```python
from build123d import *

# Parameters (mm, degrees)
SKETCH1_R           = 16
BASE_EXTRUDE_DEPTH  = 3
EXTRUDE3_DEPTH      = 62
BOSS_EXTRUDE1_DEPTH = 90
SKETCH6_R           = 16
BOSS_EXTRUDE2_DEPTH = 6
SKETCH9_W           = 18
SKETCH9_H           = 30
CUT_EXTRUDE1_DEPTH  = 107.423681603
SKETCH7_R           = 12.5
EXTRUDE4_DEPTH      = 100


with BuildPart() as part:
    # Sketch1 → Base-Extrude (new, symmetric)
    with BuildSketch(Plane.XY):
        Circle(SKETCH1_R)
    extrude(amount=BASE_EXTRUDE_DEPTH, both=True)

    # Sketch2 → Extrude3 (add)
    with BuildSketch(Plane.XY.offset(3)):
        with BuildLine():
            Line((-6, -6.5), (-6, 6.5))
            ThreePointArc((-6, 6.5), (0, 12.5), (6, 6.5))
            Line((6, 6.5), (6, -6.5))
            ThreePointArc((6, -6.5), (0, -12.5), (-6, -6.5))
        make_face()
    extrude(amount=EXTRUDE3_DEPTH)

    # Sketch5 → Boss-Extrude1 (add)
    with BuildSketch(Plane(origin=(0, 0, -3), x_dir=(-1, 0, 0), z_dir=(0, 0, -1))):
        with BuildLine():
            Line((-3, 3), (-3, 10))
            ThreePointArc((-3, 10), (0, 13), (3, 10))
            Line((3, 10), (3, 3))
            Line((3, 3), (10, 3))
            ThreePointArc((10, 3), (13, 0), (10, -3))
            Line((10, -3), (3, -3))
            Line((3, -3), (3, -10))
            ThreePointArc((3, -10), (0, -13), (-3, -10))
            Line((-3, -10), (-3, -3))
            Line((-3, -3), (-10, -3))
            ThreePointArc((-10, -3), (-13, 0), (-10, 3))
            Line((-10, 3), (-3, 3))
        make_face()
    extrude(amount=BOSS_EXTRUDE1_DEPTH)

    # Sketch6 → Boss-Extrude2 (add)
    with BuildSketch(Plane(origin=(0, 0, -93), x_dir=(-1, 0, 0), z_dir=(0, 0, -1))):
        with Locations(Location((0, 0, 0), (0, 0, 180))):
            Circle(SKETCH6_R)
    extrude(amount=BOSS_EXTRUDE2_DEPTH)

    # Sketch9 → Boss-Revolve1 (revolve)
    with BuildSketch(Plane.XY.offset(65), mode=Mode.PRIVATE) as boss_revolve1_sk:
        with Locations((0, 15)):
            Rectangle(SKETCH9_W, SKETCH9_H)
    revolve(boss_revolve1_sk.sketch.rotate(Axis((9, 0, 65), (1, 0, 0)), 180), axis=Axis((9, 0, 65), (1, 0, 0)))

    # Sketch10 → Cut-Extrude1 (cut, through all)
    with BuildSketch(Plane(origin=(9, 0, 0), x_dir=(0, 0, -1), z_dir=(1, 0, 0))):
        with BuildLine():
            Line((-72.483314774, 13), (-57.516685226, 13))
            ThreePointArc((-57.516685226, 13), (-65, -15), (-72.483314774, 13))
        make_face()
    extrude(amount=-CUT_EXTRUDE1_DEPTH, mode=Mode.SUBTRACT)

    # Sketch7 → Extrude4 (add)
    with BuildSketch(Plane(origin=(0, 0, -99), x_dir=(-1, 0, 0), z_dir=(0, 0, -1))):
        Circle(SKETCH7_R)
    extrude(amount=EXTRUDE4_DEPTH)


solid = part.part
```
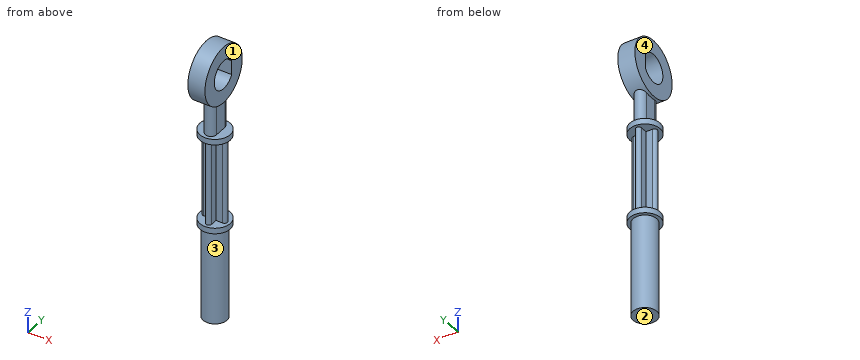
Model file for the job. Use its own axes, mm. Face numbers are marked on the shaded views. A direction names the side the tool comes from. Coordinates: 2 decimals unless noted, no trailing zeros. Write each loop counter-clockwise with the first axis right and the second up, starting at its lowest first coordinate (ties: lowest second). Pieces come first, ordered by that corner, then holes. Notation, with made-up numbers: (54.5, -37) - (103.5, -37) arc R31 ccw to (103.5, -6) - close; hole circle Ø3 at (-13, 62). An arc over 180 degrees is marked (long way). Use a Markdown table: item, result. Add a question column.
Item 1: Drop flat-ended pins along their axis: pin 1 (7.5 mm diameter, centred on x = -7, z = -58, fed in from +Y); pin 2 (18 mm diameter, centred on y = 0, z = 65, fed in from -X); pin 3 (3.5 mm diameter, centred on y = 7.5, z = -32.5, fed in from -X); pin 4 (10.5 mm diameter, centred on y = 1.5, z = 21, fed in from +X). Give the stop position or say it passes through.
Item 2: Band-saw the part on D-D, the plane y = 19. Write the cut outline in (x, z), and give its area (3 significant figures).
Item 3: Band-saw the part on A-A, the plane y = 0. Write the cut outline in (x, z), and give its area (3 significant figures).
Item 4: Band-saw the part on B-B, the plane z = -10. Write the cut outline in (x, y), and give its area (3 significant figures).
Item 5: Drill centre lines: line 1 along Z through (x, y) = (-2, 0); line 2 along Y through (x, z) = (2, 65); line 3 along Z through (x, y) = (-10, 12). Where is each one in solid material? Low to high.
Item 6: 3-axis set-ups, long thin cutter, end or side, ignore diameter. For the marked faces 1, 2, 3 and 4: which of +Z, -Z, +X, -X, +Y, -Y reach the whole face in a straight line?
Item 7: Band-saw the part on C-C, the plane z = -125.5. Write the cut outline in (x, y), and give its area (3 significant figures).
A:
| question | item | result |
|---|---|---|
| 1 | pin 1 | stops at y = 3 |
| 1 | pin 2 | passes through |
| 1 | pin 3 | stops at x = -3 |
| 1 | pin 4 | stops at x = 6 |
| 2 | outline | (-9, 41.78) - (9, 41.78) - (9, 88.22) - (-9, 88.22) - close |
| 2 | area | 836 mm² |
| 3 | outline | (-16, -99) - (-12.5, -99) - (-12.5, -199) - (12.5, -199) - (12.5, -99) - (16, -99) - (16, -93) - (13, -93) - (13, -3) - (16, -3) - (16, 3) - (6, 3) - (6, 35) - (9, 35) - (9, 50) - (-9, 50) - (-9, 35) - (-6, 35) - (-6, 3) - (-16, 3) - (-16, -3) - (-13, -3) - (-13, -93) - (-16, -93) - close; (-9, 80) - (9, 80) - (9, 95) - (-9, 95) - close |
| 3 | area | 6,150 mm² |
| 4 | outline | (-10, -3) - (-3, -3) - (-3, -10) arc R3 ccw to (3, -10) - (3, -3) - (10, -3) arc R3 ccw to (10, 3) - (3, 3) - (3, 10) arc R3 ccw to (-3, 10) - (-3, 3) - (-10, 3) arc R3 ccw to start |
| 4 | area | 261 mm² |
| 5 | line 1 | z = -199 to 50, 80 to 95 |
| 5 | line 2 | y = -30 to -15, 13 to 30 |
| 5 | line 3 | z = -99 to -93, -3 to 3 |
| 6 | face 1 | +Z, +X, +Y, -Y |
| 6 | face 2 | -Z, +X, -X, +Y, -Y |
| 6 | face 3 | -Z |
| 6 | face 4 | +Z, -X, +Y, -Y |
| 7 | outline | circle Ø25 at (0, 0) |
| 7 | area | 491 mm² |
